Verification items for the finished model (mm, model axes). A direction names the side the tool comes from. Round coordinates to 2 decimals unless told otherwise and drop trailing zeros. Loops run counter-clockwise (first coordinate to the right, second up) from the corner with the lowest first, then second, coordinate; pieces in that order, holes last.
from build123d import *

# Parameters (mm, degrees)
EXTRUDE_1_DEPTH     = 50
SKETCH_2_W          = 8.5
SKETCH_2_H          = 10.5
CUT_EXTRUDE_1_DEPTH = 52.870829554
SKETCH_3_W          = 2.75
SKETCH_3_H          = 10.5
CUT_EXTRUDE_2_DEPTH = 52.870829554
SKETCH_4_R          = 1.75
CUT_EXTRUDE_3_DEPTH = 53.975575482


with BuildPart() as part:
    # 草图1 → 凸台-拉伸1 (new body)
    with BuildSketch(Plane(origin=(0, 0, 0), x_dir=(1, 0, 0), z_dir=(0, 1, 0))):
        with BuildLine():
            Line((-8.953846154, 10.507692308), (-8.953846154, -5.492307692))
            Line((-8.953846154, -5.492307692), (3.046153846, -5.492307692))
            ThreePointArc((3.046153846, -5.492307692), (4.460367409, -4.906521255), (5.046153846, -3.492307692))
            Line((5.046153846, -3.492307692), (5.046153846, 8.507692308))
            ThreePointArc((5.046153846, 8.507692308), (4.460367409, 9.92190587), (3.046153846, 10.507692308))
            Line((3.046153846, 10.507692308), (-8.953846154, 10.507692308))
        make_face()
    extrude(amount=EXTRUDE_1_DEPTH)

    # 草图2 → 切除-拉伸1 (cut, through all)
    with BuildSketch(Plane(origin=(0, 50, 0), x_dir=(1, 0, 0), z_dir=(0, 1, 0))):
        with Locations((-1.953846154, 2.507692308)):
            Rectangle(SKETCH_2_W, SKETCH_2_H)
    extrude(amount=-CUT_EXTRUDE_1_DEPTH, mode=Mode.SUBTRACT)

    # 草图3 → 切除-拉伸2 (cut, through all)
    with BuildSketch(Plane(origin=(0, 50, 0), x_dir=(1, 0, 0), z_dir=(0, 1, 0))):
        with Locations((-7.578846154, 2.507692308)):
            Rectangle(SKETCH_3_W, SKETCH_3_H)
    extrude(amount=-CUT_EXTRUDE_2_DEPTH, mode=Mode.SUBTRACT)

    # 草图4 → 切除-拉伸3 (cut, through all)
    with BuildSketch(Plane(origin=(5.046153846, 0, 0), x_dir=(0, 0, -1), z_dir=(1, 0, 0))):
        with Locations((2.507692308, 43)):
            Circle(SKETCH_4_R)
        with Locations((2.507692308, 6)):
            Circle(SKETCH_4_R)
    extrude(amount=-CUT_EXTRUDE_3_DEPTH, mode=Mode.SUBTRACT)


solid = part.part
1. Gauge pin test, flat ends, axial feed: P1, Ø5.5, axis at y = 43, z = -2.51, coming from the -X side; P2, Ø5.5, axis at y = 6, z = -2.51, coming from the +X side; P3, Ø1.5, axis at x = 0.5, z = -0.5, coming from the +Y side. Record the tip position at first contact, or that the pin passes through.
2. Scan lines: L1, parallel to Z at x = -7.75, y = 36; L2, parallel to X at y = 16, z = 1; L3, parallel to Y at x = 4, z = -3.5. Record each from-to range of solid material in increasing order.
3. Tool access check on faces 1 (the face through (4.476, 24.65, -9.906)), 2 (the face through (-3, 25, 2.742)). Record the directions out of +Z, -Z, +X, -X, +Y, -Y that give a thin tool (end or side, any length) a straight path to the whole face; none if there is none.
4. Section check B-B (x = -4.5). Enter the section's corners in (y, z).
5. Section check C-C (y = 6). Enter the section's corners in (x, z), then the cut area to 3 significant figures.
6. Section check D-D (z = -3). Enter the section's corners in (x, y), then the cut area to 3 significant figures.
7. Release check for a two-part mould opening along Z. For faces 3 (the face through (-3, 25, -10.508)), 4 (the face through (3, 50, -4)), 5 (the face through (3.7, 4.3, -2.1)), 6 (the face through (-3, 25, 5.492)) record: released by +Z, released by -Z, zero draft, split by the parting line, or undercut.
8. Section check A-A (y = 20). Enter the section's corners in (x, z).
Taken from the geometry:
1. P1: stops at x = 2.3
1. P2: stops at x = 5.05
1. P3: passes through
2. L1: z = -10.51 to -7.76, 2.74 to 5.49
2. L2: x = 2.3 to 5.05
2. L3: y = 0 to 4.56, 7.44 to 41.56, 44.44 to 50
3. face 1: -Z, +X, +Y, -Y
3. face 2: -X, +Y, -Y
4. outline: (0, -10.51) - (50, -10.51) - (50, -7.76) - (0, -7.76) - close; (0, 2.74) - (50, 2.74) - (50, 5.49) - (0, 5.49) - close
5. outline: (-8.95, -10.51) - (3.05, -10.51) arc R2 ccw to (5.05, -8.51) - (5.05, -4.26) - (2.3, -4.26) - (2.3, -7.76) - (-8.95, -7.76) - close; (-8.95, 2.74) - (2.3, 2.74) - (2.3, -0.76) - (5.05, -0.76) - (5.05, 3.49) arc R2 ccw to (3.05, 5.49) - (-8.95, 5.49) - close
5. area: 94.5 mm2
6. outline: (2.3, 0) - (5.05, 0) - (5.05, 4.32) - (2.3, 4.32) - close; (2.3, 7.68) - (5.05, 7.68) - (5.05, 41.32) - (2.3, 41.32) - close; (2.3, 44.68) - (5.05, 44.68) - (5.05, 50) - (2.3, 50) - close
6. area: 119 mm2
7. face 3: released by -Z
7. face 4: zero draft
7. face 5: undercut
7. face 6: released by +Z
8. outline: (-8.95, -10.51) - (3.05, -10.51) arc R2 ccw to (5.05, -8.51) - (5.05, 3.49) arc R2 ccw to (3.05, 5.49) - (-8.95, 5.49) - (-8.95, 2.74) - (2.3, 2.74) - (2.3, -7.76) - (-8.95, -7.76) - close
